Design review of the part built by this model. Coordinates are the model's own, in mm. A direction names the side the tool comes from. Round coordinates to 2 decimals unless told otherwise and drop trailing zeros. Loops run counter-clockwise (first coordinate to the right, second up) from the corner with the lowest first, then second, coordinate; pieces in that order, holes last. Notation, with made-up numbers: M 44.25,-38.5 L 71.25,-38.5 A18 cw 71.25,-24.5 Z; hole C 45.5,-40 d4. An arc over 180 degrees is marked long. One line per item, written item: value. Start each with the question number.
Item 1: For line 1 along X through (y, z) = (-2.5, 40.5); line 2 along Z through (x, y) = (7, -14.5); line 3 along Z through (x, y) = (-8, -43), list the stretches that pass through material, from the lowest coordinate up.
Item 2: We need section B-B (y = -18.5). Write out the cut boundary in (x, z).
Item 3: Clearance check with flat-ended pins moving along their axes: pin 1 (20.5 mm diameter, centred on x = 10.5, z = 33, fed in from -Y); pin 2 (5 mm diameter, centred on x = 5, z = 46.5, fed in from +Y); pin 3 (12.5 mm diameter, centred on x = 8, y = -21, fed in from -Z). State where each tip first meets the part, or that it passes through.
Item 4: We need section C-C (z = 27.5). Write out the cut boundary in (x, y).
Item 5: We need section D-D (x = -7). Write out the cut boundary in (y, z), then the cut area to 3 significant figures.
Item 6: We need section A-A (x = -18). Write out the cut boundary in (y, z), then the cut area to 3 significant figures.
Item 7: Mouldability with a two-part tool opening along Z and no side actions: class faces 1 (the flat face through (-26, -25, 0)), 2 (the cylindrical face through (-28.67, -25.76, 13.06)), 3 (the flat face through (13, -22, 44.719)), 4 (the flat face through (0, -25, 14)) as released by +Z, released by -Z, zero draft, split by the parting line, or undercut.
Item 8: For faces 5 (the flat face through (-26, -36, 50.8)), 6 (the flat face through (13, -35.004, 32)), 7 (the flat face through (13, -9.604, 32)), list the 3-axis set-ups (+Z, -Z, +X, -X, +Y, -Y) from which the entire face can be reached by the end or side of a thin tool; tool diameter is ignored.
from build123d import *

# Parameters (mm, degrees)
F0_W     = 50.8
F0_H     = 50.8
F1_DEPTH = 50.8
F2_R     = 12.7
F3_DEPTH = 50.8
F4_W     = 25.4
F4_H     = 25.4
F5_DEPTH = 25.4
F6_R     = 12.7
F7_DEPTH = 25.4


with BuildPart() as f1:
    # F0 (on Front) → F1 (new body)
    with BuildSketch(Plane.XZ):
        with Locations((-25.4, 25.4)):
            Rectangle(F0_W, F0_H)
    extrude(amount=F1_DEPTH)

    # F2 (on face) → F3 (cut)
    with BuildSketch(Plane.XZ.offset(50.8)):
        with Locations((-25.91233, 25.456434)):
            Circle(F2_R)
    extrude(amount=-F3_DEPTH, mode=Mode.SUBTRACT)

    # F4 (on face) → F5 (join)
    with BuildSketch(Plane.YZ):
        with Locations((-22.304374, 32.019305)):
            Rectangle(F4_W, F4_H)
    extrude(amount=F5_DEPTH)

    # F6 (on face) → F7 (join)
    with BuildSketch(Plane.XY.offset(50.8)):
        with Locations((-26.821535, -22.958707)):
            Circle(F6_R)
    extrude(amount=F7_DEPTH)


solid = f1.part
A:
1. line 1: -50.8 to 0
1. line 2: 19.32 to 44.72
1. line 3: 0 to 50.8
2. outline: M -50.8,0 L 0,0 L 0,19.32 L 25.4,19.32 L 25.4,44.72 L 0,44.72 L 0,50.8 L -14.93,50.8 L -14.93,76.2 L -38.71,76.2 L -38.71,50.8 L -50.8,50.8 Z; hole C -25.91,25.46 d25.4
3. pin 1: y = -35
3. pin 2: y = -9.6
3. pin 3: z = 19.32
4. outline: M -50.8,-50.8 L -38.45,-50.8 L -38.45,0 L -50.8,0 Z; M -13.38,-50.8 L 0,-50.8 L 0,-35 L 25.4,-35 L 25.4,-9.6 L 0,-9.6 L 0,0 L -13.38,0 Z
5. outline: M -50.8,0 L 0,0 L 0,50.8 L -50.8,50.8 Z
5. area: 2,580 mm2
6. outline: M -50.8,0 L 0,0 L 0,15.52 L -50.8,15.52 Z; M -50.8,35.39 L 0,35.39 L 0,50.8 L -13.82,50.8 L -13.82,76.2 L -32.09,76.2 L -32.09,50.8 L -50.8,50.8 Z
6. area: 2,040 mm2
7. face 1: released by -Z
7. face 2: undercut
7. face 3: released by +Z
7. face 4: zero draft
8. face 5: +Z
8. face 6: +Z, -Z, +X, -Y
8. face 7: +Z, -Z, +X, +Y
